```python
from build123d import *

# Parameters (mm, degrees)
EXTRUDE_1_DEPTH = 5
SKETCH_2_W      = 4.503141041
SKETCH_2_H      = 8.946240201
EXTRUDE_2_DEPTH = 3


with BuildPart() as part:
    # Эскиз1 → Бобышка-Вытянуть1 (new body)
    with BuildSketch(Plane(origin=(0, 0, 0), x_dir=(1, 0, 0), z_dir=(0, 1, 0))):
        Polygon((0, 0), (11.600546573, 0), (14.80537201, 3.707393578), (14.80537201, 8.299672792), (11.09364712, 11.86425352), (5.164556962, 11.86425352), (5.164556962, 8.86425352), (9.886392586, 8.86425352), (11.80537201, 7.021348328), (11.80537201, 4.652272931), (10.218600246, 3), (0, 3), align=None)
    extrude(amount=EXTRUDE_1_DEPTH)

    # Эскиз2 → Бобышка-Вытянуть2 (add)
    with BuildSketch(Plane.ZY):
        with Locations((-1.074738625, 2.270579917)):
            Rectangle(SKETCH_2_W, SKETCH_2_H)
    extrude(amount=EXTRUDE_2_DEPTH)


solid = part.part
```
Could you check a few things on this model? Use its own coordinates, in mm. A direction names the side the tool comes from. Round coordinates to 2 decimals unless told otherwise and drop trailing zeros. Order: outer loops, then holes, each group sorted by start corner. A loop starts at its lowest first (then second) coordinate and runs counter-clockwise, first axis right, second up. Notation, with made-up numbers: M 78.25,36 L 104.25,36 A23 cw 104.25,67 Z; hole C 56,-5.75 d1. An arc over 180 degrees is marked long. One line per question, with ' | ' between items. Start each with the question number.
(1) Suppose I cut it at D-D on x = 4. List the corners of the cut face in (y, z) for me.
(2) Suppose I cut it at B-B on y = 2. List the corners of the cut face in (x, z) for me, then the cut area to 3 significant figures.
(3) Please list where these lines run through material, in increasing order: line 1 along Z through (x, y) = (8.5, 0.5); line 2 along X through (y, z) = (6.25, -2); line 3 along Y through (x, z) = (8.75, -1.5).
(4) For faces 5 (the face through (11, 0, -3)), 6 (the face through (11.805, 2, -6)), 7 (the face through (-1, 2, -3.326)), 8 (the face through (11, 5, -3)), which set-ups out of +Z, -Z, +X, -X, +Y, -Y let a thin tool reach every point of the face, with its end or its side?
(5) Suppose I cut it at A-A on x = 9. List the corners of the cut face in (y, z) for me, then the cut area to 3 significant figures.
(6) Suppose I cut it at C-C on z = -5.5. List the corners of the cut face in (x, y) for me.
(7) Thinking about a two-plate mould opening in Z: for faces 1 (the face through (12.975, 2.465, -10.057)), 2 (the face through (6, 2, 0)), 3 (the face through (5, 2, -3)), 4 (the face through (11.023, 2.465, -3.838)), which applies, +Z half, -Z half, draft (parallel to the pull), parting line (faces both ways), or undercut?
(8) For P1, Ø3, axis at x = 10.5, z = -5.5, coming from the +Y side; P2, Ø2.5, axis at x = -2, y = 1.5, coming from the -Z side; P3, Ø3.5, axis at x = 9.5, z = -5.5, coming from the -Y side; P4, Ø1, axis at y = 0, z = -4.5, coming from the -X side, each with a flat end and sliding along its axis, tell me the tip position at first contact or that it passes through.
Geometry results:
1) outline: M 0,-3 L 5,-3 L 5,0 L 0,0 Z
2) outline: M -3,-3.33 L 0,-3.33 L 0,-3 L 10.22,-3 L 11.81,-4.65 L 11.81,-7.02 L 9.89,-8.86 L 5.16,-8.86 L 5.16,-11.86 L 11.09,-11.86 L 14.81,-8.3 L 14.81,-3.71 L 11.6,0 L 0,0 L 0,1.18 L -3,1.18 Z | area: 95.0 mm²
3) line 1: -11.86 to -8.86, -3 to 0 | line 2: -3 to 0 | line 3: 0 to 5
4) face 5: +Z, -Z, +X, -Y | face 6: -X, +Y, -Y | face 7: -Z, -X, +Y, -Y | face 8: +Z, -Z, +X, +Y
5) outline: M 0,-11.86 L 5,-11.86 L 5,-8.86 L 0,-8.86 Z; M 0,-3 L 5,-3 L 5,0 L 0,0 Z | area: 30.0 mm²
6) outline: M 11.81,0 L 14.81,0 L 14.81,5 L 11.81,5 Z
7) face 1: -Z half | face 2: +Z half | face 3: undercut | face 4: undercut
8) P1: y = 5 | P2: z = -3.33 | P3: through | P4: x = 11.18
